Autodesk Inventor part; units mm, degrees
ref_plane "YZ Plane" through (0, 0, 0) normal (1, 0, 0) x (0, 1, 0)
ref_plane "XZ Plane" through (0, 0, 0) normal (0, 1, 0) x (-1, 0, 0)
ref_plane "XY Plane" through (0, 0, 0) normal (0, 0, 1) x (1, 0, 0)
sketch "Sketch1" plane through (0, 0, 0) normal (0, 1, 0) x (-1, 0, 0)
  line L0 (0, 0) -> (24, 0)
  line L1 (24, 0) -> (24, -40)
  line L2 (24, -40) -> (0, -40)
  line L3 (0, -40) -> (0, 0)
  dimension "d0" = 24
  dimension "d1" = 40
extrude "Extrusion1" add sketch "Sketch1" along normal blind 6
sketch "Sketch2" plane through (0, 6, 0) normal (0, 1, 0) x (1, 0, 0)
  arc A0 (-12, 24.25) -> (-12, 15.75) centre (-12, 20) ccw
  line L0 (-12, 15.75) -> (0, 15.75)
  line L1 (-12, 24.25) -> (0, 24.25)
  line L2 (0, 24.25) -> (0, 15.75)
  line L3 (0, 0) -> (0, 40)
  dimension "d4" = 8.5
extrude "Extrusion2" cut sketch "Sketch2" against normal blind 6
sketch "Sketch3" plane through (0, 6, 0) normal (0, 1, 0) x (1, 0, 0)
  circle A0 centre (-12, 6) radius 1.8
  point P0 (0, 0)
  dimension "d7" = 3.6
extrude "Extrusion3" cut sketch "Sketch3" against normal blind 6
ref_plane "Work Plane1" through (-24, 0, -20) normal (0, 0, 1) x (1, 0, 0)
mirror "Mirror1" about plane through (-24, 0, -20) normal (0, 0, 1) of "Extrusion3"
sketch "Sketch4" plane through (0, 0, 0) normal (0, -1, 0) x (1, 0, 0)
  circle A0 centre (-12, -6) radius 1.8
  circle A1 centre (-12, -6) radius 2.9
  point P0 (0, 0)
  dimension "d11" = 5.8
extrude "Extrusion4" cut sketch "Sketch4" against normal blind 3
mirror "Mirror2" about plane through (-24, 0, -20) normal (0, 0, 1) of "Extrusion4"
fillet "Fillet1" radius 4 6 edges at (-24, 3, -40) (0, 3, 0) (-24, 3, 0) (0, 3, -40) (0, 3, -24.25) (0, 3, -15.75)
properties part number "shaft pusher bottom"
Part model, mm, in its own coordinate system. A direction names the side the tool comes from. Coordinates: 2 decimals unless noted, no trailing zeros. Write each loop counter-clockwise with the first axis right and the second up, starting at its lowest first coordinate (ties: lowest second). Pieces come first, ordered by that corner, then holes. Notation, with made-up numbers: (54.5, 89.5) - (74.5, 89.5) arc R7 cw to (74.5, 93.5) - close; hole circle Ø3 at (-25.5, 6.5). An arc over 180 degrees is marked (long way). Put each result on its own line as item: value.
1. Band-saw the part on D-D (z = -20). Write the cut outline in (x, y).
Final values:
outline: (-24, 0) - (-16.25, 0) - (-16.25, 6) - (-24, 6) - close
2. Flat gauge pins, fed straight in: pin 1 Ø4.5 at (x, z) = (-12, -5) entering from -Y; pin 2 Ø4 at (x, z) = (-12, -34) entering from -Y; pin 3 Ø1 at (y, z) = (5, -21) entering from +X. Where does each tip first touch, or does it go through?
Final values:
pin 1: stops at y = 0
pin 2: stops at y = 3
pin 3: stops at x = -15.98
3. Two-plate mould, pull along Z, no slides. Class faces 4 (the flat face through (-12, 6, -15)), 5 (the cylindrical face through (-1.141, 3.042, -38.797)), 6 (the cylindrical face through (-14.9, 1.5, -5.9)), 7 (the cylindrical face through (-1.203, 2.958, -14.609)): +Z half, -Z half, draft (parallel to the pull), parting line (faces both ways), or undercut.
Final values:
face 4: draft
face 5: -Z half
face 6: undercut
face 7: undercut
4. 3-axis set-ups, long thin cutter, end or side, ignore diameter. For faces 1 (the flat face through (-10, 3, -6)), 2 (the flat face through (-8, 3, -15.75)), 3 (the flat face through (-24, 3, -20)): which of +Z, -Z, +X, -X, +Y, -Y reach the whole face in a straight line?
Final values:
face 1: -Y
face 2: +X, +Y, -Y
face 3: +Z, -Z, -X, +Y, -Y
5. Probe line 1 along Z through (x, y) = (-12, 5.45); line 2 along Z through (x, y) = (-12, 1.5); line 3 along X through (y, z) = (4.75, -34). List the from-to ranges inside material, lowest first. Write a range as [from, to].
Final values:
line 1: z = [-40, -35.8], [-32.2, -24.25], [-15.75, -7.8], [-4.2, 0]
line 2: z = [-40, -36.9], [-31.1, -24.25], [-15.75, -8.9], [-3.1, 0]
line 3: x = [-24, -13.8], [-10.2, 0]
6. Band-saw the part on C-C (x = -5). Write the cut outline in (y, z).
Final values:
outline: (0, -40) - (6, -40) - (6, -24.25) - (0, -24.25) - close; (0, -15.75) - (6, -15.75) - (6, 0) - (0, 0) - close
7. Band-saw the part on B-B (y = 4.4). Write the cut outline in (x, z).
Final values:
outline: (-24, -36) arc R4 ccw to (-20, -40) - (-4, -40) arc R4 ccw to (0, -36) - (0, -28.25) arc R4 ccw to (-4, -24.25) - (-12, -24.25) arc R4.25 cw to (-12, -15.75) - (-4, -15.75) arc R4 ccw to (0, -11.75) - (0, -4) arc R4 ccw to (-4, 0) - (-20, 0) arc R4 ccw to (-24, -4) - close; hole circle Ø3.6 at (-12, -34); hole circle Ø3.6 at (-12, -6)
8. Band-saw the part on A-A (z = -6). Write the cut outline in (x, y).
Final values:
outline: (-24, 0) - (-14.9, 0) - (-14.9, 3) - (-13.8, 3) - (-13.8, 6) - (-24, 6) - close; (-10.2, 3) - (-9.1, 3) - (-9.1, 0) - (0, 0) - (0, 6) - (-10.2, 6) - close
